Part model, mm, in its own coordinate system. A direction names the side the tool comes from. Coordinates: 2 decimals unless noted, no trailing zeros. Loops run counter-clockwise (first coordinate to the right, second up) from the corner with the lowest first, then second, coordinate; pieces in that order, holes last. Notation, with made-up numbers: (74, -26.5) -> (102, -26.5) arc R11 cw to (102, -12.5) -> close; hole circle Ø2 at (41, 17.25). An arc over 180 degrees is marked (long way). One line per question, with ' | ' between items. Start each with the question number.
1) Probe L1, parallel to X at y = 6.45, z = 0; L2, parallel to X at y = 1.5, z = 0; L3, parallel to Y at x = 9, z = 8. List the from-to ranges inside material, lowest first. Write a range as from..to.
2) Drop flat-ended pins along their axis: pin 1 (1 mm diameter, centred on y = 4, z = -14.5, fed in from -X); pin 2 (3 mm diameter, centred on y = 4.5, z = -4.5, fed in from +X); pin 3 (17.5 mm diameter, centred on x = 2, z = 8, fed in from -Y); pin 4 (9 mm diameter, centred on x = 0, z = 0, fed in from -Y). Give the stop position or say it passes through.
3) Cut at D-D (z = -24). List the corners of the cut face in (x, y).
4) Cut at A-A (z = 0). List the corners of the cut face in (x, y).
5) 3-axis set-ups, long thin cutter, end or side, ignore diameter. For faces 1 (the face through (-6, 8, 6)), 2 (the face through (-8, 6, 0)): which of +Z, -Z, +X, -X, +Y, -Y reach the whole face in a straight line?
6) Cut at C-C (y = 5). List the corners of the cut face in (x, z).
7) Cut at B-B (x = 0). List the corners of the cut face in (y, z), plus the area to 3 significant figures.
8) Two-plate mould, pull along X, no slides. Class faces 3 (the face through (1.32, 3.94, -29.97)), 4 (the face through (0.33, 7.014, -7.493)), 5 (the face through (-13, 0, 13)): released by +X, released by -X, zero draft, split by the parting line, or undercut.
from build123d import *

# Parameters (mm, degrees)
ESQUISSE1_R             = 30
BOSS_EXTRU_1_DEPTH      = 8
ESQUISSE2_R             = 17.5
ENL_V_MAT_EXTRU_1_DEPTH = 6
ESQUISSE3_R             = 7.5
ENL_V_MAT_EXTRU_2_DEPTH = 44.17406629


with BuildPart() as part:
    # Esquisse1 → Boss.-Extru.1 (new body)
    with BuildSketch(Plane(origin=(0, 0, 0), x_dir=(1, 0, 0), z_dir=(0, 1, 0))):
        with Locations(Location((0, 0, 0), (0, 0, 270))):
            Circle(ESQUISSE1_R)
    extrude(amount=BOSS_EXTRU_1_DEPTH)

    # Esquisse2 → Enlèv. mat.-Extru.1 (cut)
    with BuildSketch(Plane.XZ):
        with Locations(Location((0, 0, 0), (0, 0, 270))):
            Circle(ESQUISSE2_R)
    extrude(amount=-ENL_V_MAT_EXTRU_1_DEPTH, mode=Mode.SUBTRACT)

    # Esquisse3 → Enlèv. mat.-Extru.2 (cut, through all)
    with BuildSketch(Plane(origin=(0, 8, 0), x_dir=(1, 0, 0), z_dir=(0, 1, 0))):
        with Locations(Location((0, 0, 0), (0, 0, 270))):
            Circle(ESQUISSE3_R)
    extrude(amount=-ENL_V_MAT_EXTRU_2_DEPTH, mode=Mode.SUBTRACT)


solid = part.part
Reported:
1) L1: x = -30..-7.5, 7.5..30 | L2: x = -30..-17.5, 17.5..30 | L3: y = 6..8
2) pin 1: stops at x = -26.53 | pin 2: stops at x = 29.85 | pin 3: stops at y = 6 | pin 4: passes through
3) outline: (-18, 0) -> (18, 0) -> (18, 8) -> (-18, 8) -> close
4) outline: (-30, 0) -> (-17.5, 0) -> (-17.5, 6) -> (-7.5, 6) -> (-7.5, 8) -> (-30, 8) -> close; (7.5, 6) -> (17.5, 6) -> (17.5, 0) -> (30, 0) -> (30, 8) -> (7.5, 8) -> close
5) face 1: +Z, -Z, +X, -X, +Y | face 2: -Y
6) outline: circle Ø60 at (0, 0); hole circle Ø35 at (0, 0)
7) outline: (0, -30) -> (8, -30) -> (8, -7.5) -> (6, -7.5) -> (6, -17.5) -> (0, -17.5) -> close; (0, 17.5) -> (6, 17.5) -> (6, 7.5) -> (8, 7.5) -> (8, 30) -> (0, 30) -> close | area: 240 mm²
8) face 3: split by the parting line | face 4: undercut | face 5: zero draft
